Design review of the part built by this model. Coordinates are the model's own, in mm. A direction names the side the tool comes from. Give positions to 0.01 mm unless a question says otherwise; leave off trailing zeros. Loops run counter-clockwise (first coordinate to the right, second up) from the corner with the lowest first, then second, coordinate; pieces in that order, holes last. Notation, with made-up numbers: M 31,54 L 66,54 A30 cw 66,76 Z; hole C 77.5,-38 d10. An arc over 180 degrees is marked long. Answer as CSV lines item,"result".
```python
from build123d import *

# Parameters (mm, degrees)
SKETCH1_W                          = 65
SKETCH1_H                          = 38
BOSS_EXTRUDE1_DEPTH                = 22
SKETCH2_W                          = 82
SKETCH2_H                          = 10
BOSS_EXTRUDE2_DEPTH                = 2
F_3_0_3_DIAMETER_HOLE1_D           = 3
F_3_0_3_DIAMETER_HOLE1_CSINK_D     = 3.05
F_3_0_3_DIAMETER_HOLE1_CSINK_ANGLE = 90


with BuildPart() as part:
    # Sketch1 → Boss-Extrude1 (new body)
    with BuildSketch(Plane(origin=(0, 0, 0), x_dir=(1, 0, 0), z_dir=(0, 1, 0))):
        Rectangle(SKETCH1_W, SKETCH1_H)
    extrude(amount=BOSS_EXTRUDE1_DEPTH)

    # Sketch2 → Boss-Extrude2 (add)
    with BuildSketch(Plane.XZ):
        Rectangle(SKETCH2_W, SKETCH2_H)
    extrude(amount=-BOSS_EXTRUDE2_DEPTH)

    # Ø3.0 (3) Diameter Hole1 (through all)
    with Locations(Plane(origin=(0, 2, 0), x_dir=(1, 0, 0), z_dir=(0, 1, 0))):
        with Locations((-36.5, 0), (36.5, 0)):
            CounterSinkHole(F_3_0_3_DIAMETER_HOLE1_D / 2, F_3_0_3_DIAMETER_HOLE1_CSINK_D / 2, counter_sink_angle=F_3_0_3_DIAMETER_HOLE1_CSINK_ANGLE)


solid = part.part
```
1. For P1, Ø2.5, axis at x = 36.5, z = 0, coming from the +Y side; P2, Ø1.5, axis at y = 17, z = -3, coming from the +X side; P3, Ø2, axis at x = 38, y = 1, coming from the -Z side; P4, Ø1, axis at x = 38, y = 1, coming from the +Z side, all flat-tipped, find the tip position at first contact; note any pin that passes through.
Answer block:
P1,"through"
P2,"x = 32.5"
P3,"z = -5"
P4,"z = 5"
2. For faces 1 (the flat face through (37, 1, 5)), 2 (the flat face through (37, 1, -5)), 3 (the flat face through (-38, 2, -1)), list the 3-axis set-ups (+Z, -Z, +X, -X, +Y, -Y) from which the entire face can be reached by the end or side of a thin tool; tool diameter is ignored.
Answer block:
face 1,"+Z, +X, +Y, -Y"
face 2,"-Z, +X, +Y, -Y"
face 3,"+Z, -Z, -X, +Y"
3. To check wall thickness, follow L1, parallel to Z at x = 36.5, y = 1.15; L2, parallel to X at y = 1.5, z = -7.5; L3, parallel to Z at x = -33.5, y = 1.5. State the ranges of each line that lie inside material, in increasing order. Write a range as [from, to].
Answer block:
L1,"[-5, -1.5], [1.5, 5]"
L2,"[-32.5, 32.5]"
L3,"[-5, 5]"
4. The part is to be moulded in two halves that separate along X. For faces 4 (the flat face through (38, 2, 1)), 5 (the flat face through (-41, 1, 0)), 6 (the cylindrical face through (37.7, 1, 0.9)), say which applies: pulls with the +X half, pulls with the -X half, needs draft (parallel to the pull), parting line crosses it, or undercut.
Answer block:
face 4,"needs draft"
face 5,"pulls with the -X half"
face 6,"undercut"
5. We need section D-D, the plane z = -10.5. Write out the cut boundary in (x, y).
Answer block:
outline,"M -32.5,0 L 32.5,0 L 32.5,22 L -32.5,22 Z"
6. We need section C-C, the plane y = 5.5. Write out the cut boundary in (x, z).
Answer block:
outline,"M -32.5,-19 L 32.5,-19 L 32.5,19 L -32.5,19 Z"
7. We need section A-A, the plane x = 36.5. Write out the cut boundary in (y, z) (3 decimals).
Answer block:
outline,"M 0,-5 L 2,-5 L 2,-1.525 L 1.975,-1.5 L 0,-1.5 Z; M 0,1.5 L 1.975,1.5 L 2,1.525 L 2,5 L 0,5 Z"
8. We need section B-B, the plane z = 0. Write out the cut boundary in (x, y) (3 decimals).
Answer block:
outline,"M -41,0 L -38,0 L -38,1.975 L -38.025,2 L -41,2 Z; M -35,0 L 35,0 L 35,1.975 L 34.975,2 L 32.5,2 L 32.5,22 L -32.5,22 L -32.5,2 L -34.975,2 L -35,1.975 Z; M 38,0 L 41,0 L 41,2 L 38.025,2 L 38,1.975 Z"
